Drawing for the job (mm, zero at the part's lowest x, y, z). A direction names the side the tool comes from. Round coordinates to 2 decimals unless told otherwise and drop trailing zeros. Write each loop counter-clockwise with the first axis right and the second up, starting at its lowest first coordinate (ties: lowest second). Pieces come first, ordered by that corner, then holes.
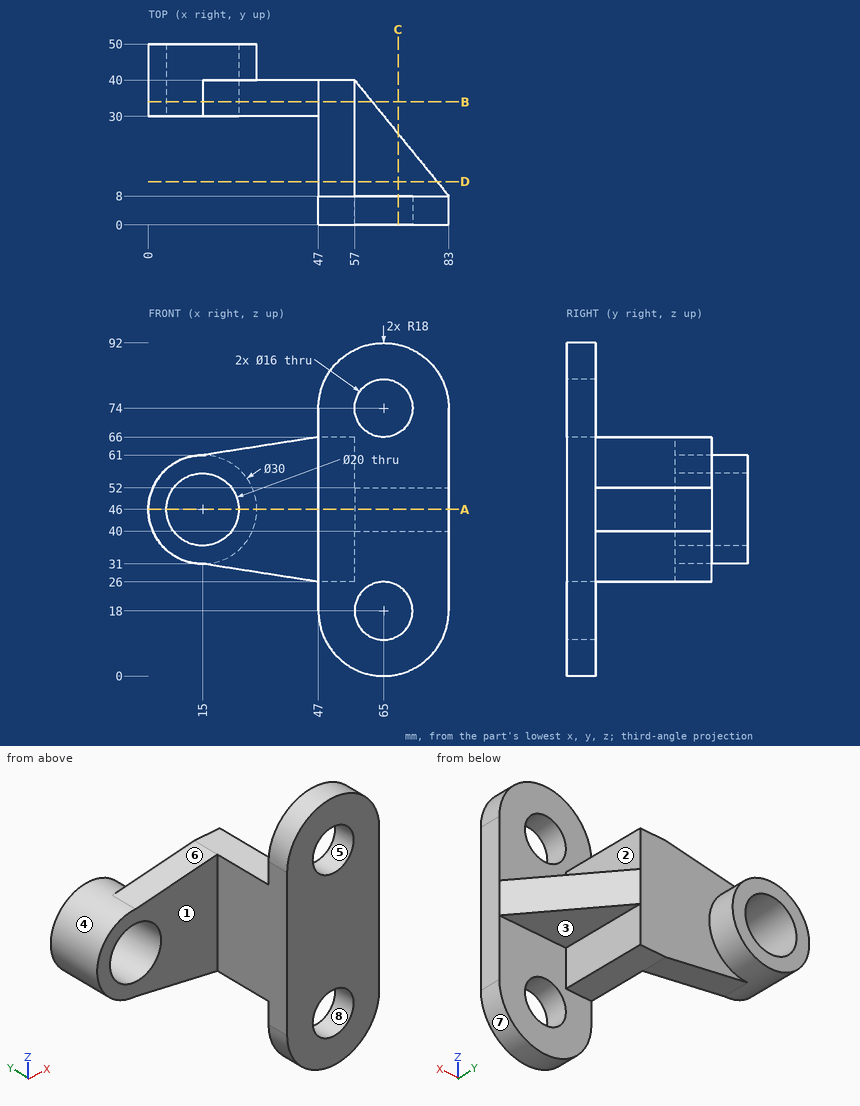
Q1. Two-plate mould, pull along X, no slides. Class the marked faces 5, 6, 7 and 8: released by +X, released by -X, zero draft, split by the parting line, or undercut.
Q2. Drop flat-ended pins along their axis: P1, Ø4, axis at y = 29, z = 66, coming from the +X side; P2, Ø18, axis at x = 60, z = 26, coming from the +Y side; P3, Ø12, axis at x = 68.5, y = 33.5, coming from the +Z side; P4, Ø24, axis at y = 19.5, z = 46.5, coming from the -X side. Give the stop position or say it passes through.
Q3. Saw through at D-D, the plane y = 12. Write the cut outline in (x, z), and give its area (3 significant figures).
Q4. Saw through at B-B, the plane y = 34. Write the cut outline in (x, z) (3 decimals), and give its area (3 significant figures).
Q5. Tool access for the marked faces 1, 2, 3 and 4: list every direction of +Z, -Z, +X, -X, +Y, -Y with a clear straight run to the whole face (end or side of a thin tool).
Q6. Saw through at A-A, the plane z = 46. Write the cut outline in (x, y), and give its area (3 significant figures).
Q7. Wall check: line 1 (Z direction, x = 65, y = 5); line 2 (X direction, y = 2, z = 18); line 3 (Z direction, x = 7, y = 35.5). Give the ranges that are in metal, low to high.
Q8. Saw through at C-C, the plane x = 69. Write the cut outline in (y, z), and give its area (3 significant figures).
Computed:
1. face 5: undercut
1. face 6: released by -X
1. face 7: split by the parting line
1. face 8: undercut
2. P1: stops at x = 57
2. P2: stops at y = 40
2. P3: stops at z = 52
2. P4: stops at x = 0
3. outline: (47, 26) - (57, 26) - (57, 40) - (79.75, 40) - (79.75, 52) - (57, 52) - (57, 66) - (47, 66) - close
3. area: 673 mm2
4. outline: (15, 31) - (47, 26) - (57, 26) - (57, 40) - (61.875, 40) - (61.875, 52) - (57, 52) - (57, 66) - (47, 66) - (15, 61) arc R15 ccw to start; hole circle Ø20 at (15, 46)
4. area: 1,620 mm2
5. face 1: +Z, -Z, -X, -Y
5. face 2: +Z, +X, +Y
5. face 3: -Z, +X, +Y
5. face 4: +Y
6. outline: (0, 30) - (5, 30) - (5, 50) - (0, 50) - close; (25, 30) - (47, 30) - (47, 0) - (83, 0) - (83, 8) - (57, 40) - (30, 40) - (30, 50) - (25, 50) - close
6. area: 1,390 mm2
7. line 1: z = 0 to 10, 26 to 66, 82 to 92
7. line 2: x = 47 to 57, 73 to 83
7. line 3: z = 33.31 to 40, 52 to 58.69
8. outline: (0, 0.45) - (8, 0.45) - (8, 11.07) - (0, 11.07) - close; (0, 24.93) - (8, 24.93) - (8, 40) - (25.23, 40) - (25.23, 52) - (8, 52) - (8, 67.07) - (0, 67.07) - close; (0, 80.93) - (8, 80.93) - (8, 91.55) - (0, 91.55) - close
8. area: 714 mm2
